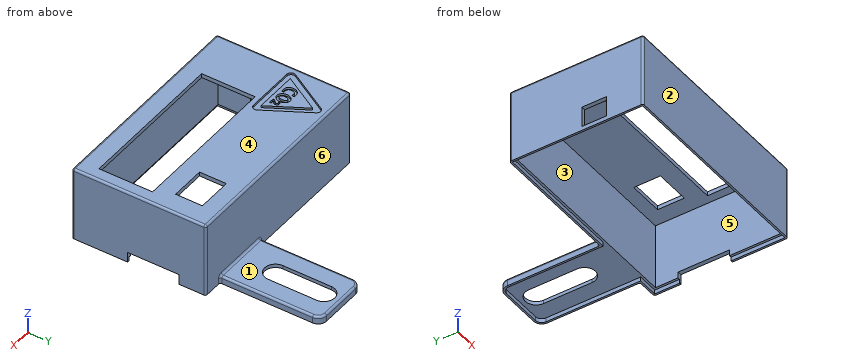
```python
from build123d import *

# Parameters (mm, degrees)
CROQUIS1_W              = 103
CROQUIS1_H              = 65
SALIENTE_EXTRUIR2_DEPTH = 36
VACIADO7_T              = -2
CORTAR_EXTRUIR28_REACH  = 73.683
CROQUIS12_W             = 73
CROQUIS12_H             = 26
SALIENTE_EXTRUIR3_DEPTH = 3.75
CORTAR_EXTRUIR11_DEPTH  = 2
CORTAR_EXTRUIR17_REACH  = 137.001
CROQUIS16_W             = 10
CROQUIS16_H             = 12
CORTAR_EXTRUIR29_REACH  = 103.334
CROQUIS30_W             = 17
CROQUIS30_H             = 13
CROQUIS20_RX            = 3.244161213
CROQUIS20_RY            = 2.649478984
CROQUIS20_RX_2          = 2.029667585
CROQUIS20_RY_2          = 1.104878059
CORTAR_EXTRUIR24_DEPTH  = 1
CORTAR_EXTRUIR30_REACH  = 137.001
CROQUIS31_W             = 5
CROQUIS31_H             = 25
REDONDEO1_R             = 1


with BuildPart() as part:
    # Croquis1 → Saliente-Extruir2 (new body)
    with BuildSketch(Plane.XY):
        with Locations((0, -2)):
            Rectangle(CROQUIS1_W, CROQUIS1_H)
    extrude(amount=SALIENTE_EXTRUIR2_DEPTH)

    # Vaciado7
    vaciado7_openings = [part.faces().sort_by_distance(p)[0] for p in [
        (0, -2, 0),
    ]]
    offset(amount=VACIADO7_T, openings=vaciado7_openings, kind=Kind.INTERSECTION)

    # Croquis12 → Cortar-Extruir28 (cut, up to next)
    with BuildSketch(Plane.XY.offset(36), mode=Mode.PRIVATE) as cortar_extruir28_sk1:
        with Locations((9, -12.5)):
            Rectangle(CROQUIS12_W, CROQUIS12_H)
    cortar_extruir28_tool1 = extrude(cortar_extruir28_sk1.sketch, amount=-CORTAR_EXTRUIR28_REACH, mode=Mode.PRIVATE) & part.part
    add(cortar_extruir28_tool1.solids().sort_by_distance((9, -12.5, 36))[0], mode=Mode.SUBTRACT)

    # Croquis29 → Saliente-Extruir3 (add)
    with BuildSketch(Plane(origin=(0, 0, 0), x_dir=(-1, 0, 0), z_dir=(0, 0, -1))):
        with BuildLine():
            Line((-13, 75.5), (-13, 30.5))
            Line((-13, 30.5), (-41.5, 30.5))
            Line((-41.5, 30.5), (-41.5, 75.5))
            ThreePointArc((-41.5, 75.5), (-40.328427125, 78.328427125), (-37.5, 79.5))
            Line((-37.5, 79.5), (-17, 79.5))
            ThreePointArc((-17, 79.5), (-14.171572875, 78.328427125), (-13, 75.5))
        make_face()
        with BuildLine():
            Line((-22, 71.25), (-22, 47.75))
            ThreePointArc((-22, 47.75), (-27.25, 42.5), (-32.5, 47.75))
            Line((-32.5, 47.75), (-32.5, 71.25))
            ThreePointArc((-32.5, 71.25), (-27.25, 76.5), (-22, 71.25))
        make_face(mode=Mode.SUBTRACT)
    extrude(amount=-SALIENTE_EXTRUIR3_DEPTH)

    # Croquis14 → Cortar-Extruir11 (cut)
    with BuildSketch(Plane(origin=(0, 0, 0), x_dir=(-1, 0, 0), z_dir=(0, 0, -1))):
        with BuildLine():
            Line((50.6, -33.6), (50.6, 29.6))
            Line((50.6, 29.6), (-13.9, 29.6))
            Line((-13.9, 29.6), (-13.9, 75.5))
            ThreePointArc((-13.9, 75.5), (-14.807968978, 77.692031022), (-17, 78.6))
            Line((-17, 78.6), (-37.5, 78.6))
            ThreePointArc((-37.5, 78.6), (-39.692031022, 77.692031022), (-40.6, 75.5))
            Line((-40.6, 75.5), (-40.6, 29.6))
            Line((-40.6, 29.6), (-50.6, 29.6))
            Line((-50.6, 29.6), (-50.6, -33.6))
            Line((-50.6, -33.6), (50.6, -33.6))
        make_face()
    extrude(amount=-CORTAR_EXTRUIR11_DEPTH, mode=Mode.SUBTRACT)

    # Croquis16 → Cortar-Extruir17 (cut, up to next)
    with BuildSketch(Plane.ZY.offset(51.5), mode=Mode.PRIVATE) as cortar_extruir17_sk1:
        with Locations((7, -10.75)):
            Rectangle(CROQUIS16_W, CROQUIS16_H)
    cortar_extruir17_tool1 = extrude(cortar_extruir17_sk1.sketch, amount=-CORTAR_EXTRUIR17_REACH, mode=Mode.PRIVATE) & part.part
    add(cortar_extruir17_tool1.solids().sort_by_distance((-51.5, -10.75, 7))[0], mode=Mode.SUBTRACT)

    # Croquis30 → Cortar-Extruir29 (cut, up to next)
    with BuildSketch(Plane.XY.offset(36), mode=Mode.PRIVATE) as cortar_extruir29_sk1:
        with Locations((33, 15.5)):
            Rectangle(CROQUIS30_W, CROQUIS30_H)
    cortar_extruir29_tool1 = extrude(cortar_extruir29_sk1.sketch, amount=-CORTAR_EXTRUIR29_REACH, mode=Mode.PRIVATE) & part.part
    add(cortar_extruir29_tool1.solids().sort_by_distance((33, 15.5, 36))[0], mode=Mode.SUBTRACT)

    # Croquis20 → Cortar-Extruir24 (cut)
    # profile 1 of 4: a face of its own
    with BuildSketch(Plane.XY.offset(36)):
        with BuildLine():
            Line((-32.877371929, 26.422410606), (-21.038034651, 5.891314445))
            ThreePointArc((-21.038034651, 5.891314445), (-21.038818093, 3.891767038), (-22.770607635, 2.892219426))
            Line((-22.770607635, 2.892219426), (-46.505903571, 2.892219426))
            ThreePointArc((-46.505903571, 2.892219426), (-48.238726232, 3.89355751), (-48.236407571, 5.894893803))
            Line((-48.236407571, 5.894893803), (-36.340448913, 26.425989964))
            ThreePointArc((-36.340448913, 26.425989964), (-34.607877759, 27.423314519), (-32.877371929, 26.422410606))
        make_face()
        Polygon((-24.134944502, 5.589013553), (-44.975333507, 5.589013553), (-34.530281265, 23.61600727), align=None, mode=Mode.SUBTRACT)
    # profile 2 of 4: a face of its own
    with BuildSketch(Plane.XY.offset(36)):
        with BuildLine():
            add(Edge.make_bspline(
                [(-36.492042346, 12.163564203), (-36.721798149, 12.216584773), (-36.946159791, 12.305207397), (-37.181309753, 12.322625912), (-37.428691713, 12.340950502), (-37.677714014, 12.302389838), (-37.92359773, 12.269605343), (-39.211705056, 12.097857699), (-39.130223403, 10.008481597), (-38.824947416, 9.194412297), (-38.471289709, 8.251325078), (-37.239201594, 8.380618349), (-36.492042346, 8.50514489)],
                knots=[0, 0, 0, 0, 1, 1, 1, 2, 2, 2, 3, 3, 3, 4, 4, 4, 4], degree=3))
            Line((-36.492042346, 8.50514489), (-36.386001207, 7.338692355))
            add(Edge.make_bspline(
                [(-36.386001207, 7.338692355), (-37.455699366, 7.204980085), (-38.280952684, 7.103931885), (-39.249111974, 7.550774634), (-39.294499295, 7.571722629), (-39.319806067, 7.621468727), (-39.355153113, 7.656815774), (-39.704014417, 8.005677078), (-40.006289411, 8.220522758), (-40.203482229, 8.664206599), (-40.972994564, 10.395609351), (-40.466643717, 12.540322436), (-38.665885706, 13.276996168), (-37.884767663, 13.596544459), (-37.05562877, 13.587263649), (-36.279960067, 13.276996168)],
                knots=[0, 0, 0, 0, 1, 1, 1, 2, 2, 2, 3, 3, 3, 4, 4, 4, 5, 5, 5, 5], degree=3))
            Line((-36.279960067, 13.276996168), (-36.492042346, 12.163564203))
        make_face()
    # profile 3 of 4: a face of its own
    with BuildSketch(Plane.XY.offset(36)):
        with Locations(Location((-33.188828288, 10.362256285), (0, 0, -90.640192277))):
            Ellipse(CROQUIS20_RX, CROQUIS20_RY)
        with Locations(Location((-33.20228715, 10.364336342), (0, 0, -89.299840613))):
            Ellipse(CROQUIS20_RX_2, CROQUIS20_RY_2, mode=Mode.SUBTRACT)
    # profile 4 of 4: a face of its own
    with BuildSketch(Plane.XY.offset(36)):
        with BuildLine():
            add(Edge.make_bspline(
                [(-30.341656255, 7.232651216), (-30.323982731, 7.462407018), (-30.379408301, 7.710115851), (-30.288635685, 7.921918623), (-30.185338507, 8.162945371), (-27.605603956, 10.360864831), (-29.440306569, 10.360864831), (-29.809630445, 10.360864831), (-29.823242351, 10.225365458), (-30.129573976, 10.148782552)],
                knots=[0, 0, 0, 0, 1, 1, 1, 2, 2, 2, 3, 3, 3, 3], degree=3))
            Line((-30.129573976, 10.148782552), (-30.341656255, 10.785029389))
            add(Edge.make_bspline(
                [(-30.341656255, 10.785029389), (-28.897370629, 11.507172202), (-27.775654694, 11.154718258), (-28.008751185, 9.406494576), (-28.069313134, 8.952279958), (-28.865628872, 8.254816587), (-29.12218315, 7.974939192)],
                knots=[0, 0, 0, 0, 1, 1, 1, 2, 2, 2, 2], degree=3))
            Line((-29.12218315, 7.974939192), (-27.84858536, 7.974939192))
            Line((-27.84858536, 7.974939192), (-27.84858536, 7.230680553))
            Line((-27.84858536, 7.230680553), (-30.341656255, 7.232651216))
        make_face()
    extrude(amount=-CORTAR_EXTRUIR24_DEPTH, mode=Mode.SUBTRACT)

    # Croquis31 → Cortar-Extruir30 (cut, up to next)
    with BuildSketch(Plane(origin=(51.5, 0, 0), x_dir=(0, 0, -1), z_dir=(1, 0, 0)), mode=Mode.PRIVATE) as cortar_extruir30_sk1:
        with Locations((-2.5, 5)):
            Rectangle(CROQUIS31_W, CROQUIS31_H)
    cortar_extruir30_tool1 = extrude(cortar_extruir30_sk1.sketch, amount=-CORTAR_EXTRUIR30_REACH, mode=Mode.PRIVATE) & part.part
    add(cortar_extruir30_tool1.solids().sort_by_distance((51.5, 5, 2.5))[0], mode=Mode.SUBTRACT)

    # Redondeo1
    redondeo1_edges = [part.edges().sort_by_distance(p)[0] for p in [
        (51.5, -2, 36),
        (0, 30.5, 36),
        (40.328427125, 78.328427125, 3.75),
        (27.25, 79.5, 3.75),
        (14.171572875, 78.328427125, 3.75),
        (13, 53, 3.75),
        (27.25, 30.5, 3.75),
        (13, 30.5, 1.875),
        (41.5, 53, 3.75),
        (41.5, 30.5, 1.875),
        (-51.5, -2, 36),
        (-51.5, 30.5, 18),
        (51.5, 30.5, 18),
        (51.5, -34.5, 18),
        (-51.5, -34.5, 18),
        (0, -34.5, 36),
    ]]
    fillet(redondeo1_edges, radius=REDONDEO1_R)


solid = part.part
```
Design review of the part built by this model. Coordinates are the model's own, in mm. Face numbers are marked on the shaded views. A direction names the side the tool comes from. Give positions to 0.01 mm unless a question says otherwise; leave off trailing zeros. Loops run counter-clockwise (first coordinate to the right, second up) from the corner with the lowest first, then second, coordinate; pieces in that order, holes last. Notation, with made-up numbers: M 33.25,-8.75 L 61.25,-8.75 A31 ccw 61.25,27.25 Z; hole C 38,84.5 d11. An arc over 180 degrees is marked long. Return JSON: item names as keys, results as strings. Group by question number.
Item 1: We need section D-D (x = 27.25). Give the number of separate pieces and of enclosed holes in the cut face, and give its area (3 significant figures).
Item 2: Tool access review of the marked faces 1, 2 and 3: name each direction out of +Z, -Z, +X, -X, +Y, -Y from which nothing blocks a thin tool from reaching the whole face with its end or side.
Item 3: We need section C-C (y = -12). Give the boundary of the cut face in (x, z), and give its area (3 significant figures).
Item 4: We need section A-A (x = 44). Give the boundary of the cut face in (y, z).
Item 5: We need section B-B (z = 24.5). Give the boundary of the cut face in (x, y), and give its area (3 significant figures).
Item 6: Insertion check: pin 1 Ø1 at (x, z) = (50.5, 3) entering from +Y; pin 2 Ø0.8 at (x, z) = (-38.5, 35.5) entering from -Y (3 decimals); pin 3 Ø13 at (x, y) = (-16.5, -27) entering from -Z. Each pin has a flat end and moves straight along its axis. Give the tip position at first contact, or say it passes through.
Item 7: For probe 1 along X at (y, z) = (7, 13); probe 2 along Y at (x, z) = (33.5, 19); probe 3 along Y at (x, z) = (3, 34.5), list the stretches that pass through material, from the lowest coordinate up.
Item 8: Mouldability with a two-part tool opening along Y and no side actions: class the marked faces 4, 5 and 6 as released by +Y, released by -Y, zero draft, split by the parting line, or undercut.
Output:
{
 "1": {"separate pieces": "4", "enclosed holes": "0", "area": "209 mm^2"},
 "2": {"face 1": "+Z, +X, -X, +Y", "face 2": "+Z, -Z, +X, -X, -Y", "face 3": "-Z"},
 "3": {"outline": "M -51.5,0 L -50.6,0 L -50.6,2 L -51.5,2 Z; M -51.5,12 L -49.5,12 L -49.5,34 L -27.5,34 L -27.5,36 L -50.5,36 A1 ccw -51.5,35 Z; M 45.5,34 L 49.5,34 L 49.5,2 L 50.6,2 L 50.6,0 L 51.5,0 L 51.5,35 A1 ccw 50.5,36 L 45.5,36 Z", "area": "171 mm^2"},
 "4": {"outline": "M -34.5,0 L -33.6,0 L -33.6,2 L -32.5,2 L -32.5,34 L -25.5,34 L -25.5,36 L -33.5,36 A1 ccw -34.5,35 Z; M 0.5,34 L 28.5,34 L 28.5,2 L 29.6,2 L 29.6,0 L 30.5,0 L 30.5,35 A1 ccw 29.5,36 L 0.5,36 Z"},
 "5": {"outline": "M -51.5,-33.5 A1 ccw -50.5,-34.5 L 50.5,-34.5 A1 ccw 51.5,-33.5 L 51.5,29.5 A1 ccw 50.5,30.5 L -50.5,30.5 A1 ccw -51.5,29.5 Z; hole M -49.5,-32.5 L 49.5,-32.5 L 49.5,28.5 L -49.5,28.5 Z", "area": "655 mm^2"},
 "6": {"pin 1": "stops at y = 30.5", "pin 2": "stops at y = -34.495", "pin 3": "stops at z = 2"},
 "7": {"probe 1": "x = -51.5 to -49.5, 49.5 to 51.5", "probe 2": "y = -34.5 to -32.5, 28.5 to 30.5", "probe 3": "y = -34.5 to -25.5, 0.5 to 30.5"},
 "8": {"face 4": "zero draft", "face 5": "undercut", "face 6": "released by +Y"}
}
